Verification items for the finished model (mm, model axes). A direction names the side the tool comes from. Give positions to 0.01 mm unless a question says otherwise; leave off trailing zeros. Order: outer loops, then holes, each group sorted by start corner. A loop starts at its lowest first (then second) coordinate and runs counter-clockwise, first axis right, second up.
(1) Scan lines: L1, parallel to X at y = 16, z = -186; L2, parallel to Z at x = 152, y = 9.5; L3, parallel to Y at x = 197, z = -14. Record each from-to range of solid material in increasing order.
(2) Mould release check, pull along Y, two halves, no side actions. Record for faces 1 (the face through (44.071, 30, -186)), 2 (the face through (46.576, 52.068, -185.846)), 3 (the face through (67.531, 25.555, -11.772)): pulls with the +Y half, pulls with the -Y half, needs draft (parallel to the pull), parting line crosses it, or undercut.
(3) Gauge pin test, flat ends, axial feed: pin 1 (9.5 mm diameter, centred on y = 20.5, z = -8, fed in from +X); pin 2 (2 mm diameter, centred on x = 216, z = -131.5, fed in from +Y); pin 3 (6 mm diameter, centred on y = 42.545, z = -186.055, fed in from -X); pin 4 (1.5 mm diameter, centred on x = 122.5, y = 14, fed in from -Z). Record the tip position at first contact, or that the pin passes through.
(4) Sectioned sample at B-B on z = -138. Record the cut outline in (x, y).
(5) Access from +Z, -Z, +X, -X, +Y, -Y to the whole of each face (thin tool, end or side, straight path). Record for faces 4 (the face through (67.531, 33.018, -9.316)), 5 (the face through (70.106, 20, -9)), 6 (the face through (46.576, 41.28, -183.005)), 7 (the face through (153.672, 30, -186)), 8 (the face through (156.466, 20, -9)).
(6) Sectioned sample at A-A on x = 246.5. Record the cut outline in (y, z), plus the area to 3 significant figures.
```python
from build123d import *

# Parameters (mm, degrees)
SKETCH1_W               = 342.9
SKETCH1_H               = 195.58
BOSS_EXTRUDE1_DEPTH     = 7.62
SKETCH2_W               = 5.08
SKETCH2_H               = 19.05
BOSS_EXTRUDE2_DEPTH     = 25.4
SKETCH3_R               = 3.048
CUT_EXTRUDE1_DEPTH      = 309.353685576
SKETCH2_4_W             = 5.08
SKETCH2_4_H             = 19.05
SKETCH2_4_W_2           = 9.525
BOSS_EXTRUDE3_DEPTH     = 44.45
SKETCH4_R               = 3.302
CUT_EXTRUDE2_DEPTH      = 45.071314424
CUT_EXTRUDE2_DEPTH_BACK = 492.252


with BuildPart() as part:
    # Sketch1 → Boss-Extrude1 (new body)
    with BuildSketch(Plane(origin=(0, 0, 0), x_dir=(1, 0, 0), z_dir=(0, 1, 0))):
        with Locations((171.45, 97.79)):
            Rectangle(SKETCH1_W, SKETCH1_H)
    extrude(amount=BOSS_EXTRUDE1_DEPTH)

    # Sketch2 → Boss-Extrude2 (add)
    with BuildSketch(Plane(origin=(0, 7.62, 0), x_dir=(1, 0, 0), z_dir=(0, 1, 0))):
        with Locations((37.086314424, 9.525)):
            Rectangle(SKETCH2_W, SKETCH2_H)
        with Locations((67.566314424, 9.525)):
            Rectangle(SKETCH2_W, SKETCH2_H)
        with Locations((153.926314424, 9.525)):
            Rectangle(SKETCH2_W, SKETCH2_H)
        with Locations((123.446314424, 9.525)):
            Rectangle(SKETCH2_W, SKETCH2_H)
    extrude(amount=BOSS_EXTRUDE2_DEPTH)

    # Sketch3 → Cut-Extrude1 (cut, through all)
    with BuildSketch(Plane.ZY.offset(-34.546314424)):
        with Locations((-9.525, 23.495)):
            Circle(SKETCH3_R)
        with BuildLine():
            Line((-19.05, 23.495), (-20.422011891, 33.02))
            Line((-20.422011891, 33.02), (2.969055393, 35.880507904))
            Line((2.969055393, 35.880507904), (0, 23.495))
            ThreePointArc((0, 23.495), (-9.525, 33.02), (-19.05, 23.495))
        make_face()
    extrude(amount=-CUT_EXTRUDE1_DEPTH, mode=Mode.SUBTRACT)

    # Sketch2_4 → Boss-Extrude3 (add)
    with BuildSketch(Plane(origin=(0, 7.62, 0), x_dir=(1, 0, 0), z_dir=(0, 1, 0))):
        with Locations((46.611314424, 186.055)):
            Rectangle(SKETCH2_4_W, SKETCH2_4_H)
        with Locations((98.871814424, 186.055)):
            Rectangle(SKETCH2_4_W_2, SKETCH2_4_H)
        with Locations((151.132314424, 186.055)):
            Rectangle(SKETCH2_4_W, SKETCH2_4_H)
    extrude(amount=BOSS_EXTRUDE3_DEPTH)

    # Sketch4 → Cut-Extrude2 (cut, two sides)
    with BuildSketch(Plane.ZY.offset(-44.071314424)) as cut_extrude2_sk:
        with Locations((-186.055, 42.545)):
            Circle(SKETCH4_R)
        with BuildLine():
            Line((-195.58, 42.545), (-197.59428292, 55.074082425))
            Line((-197.59428292, 55.074082425), (-172.116639762, 54.451508438))
            Line((-172.116639762, 54.451508438), (-176.53, 42.545))
            ThreePointArc((-176.53, 42.545), (-186.055, 52.07), (-195.58, 42.545))
        make_face()
    extrude(amount=CUT_EXTRUDE2_DEPTH, mode=Mode.SUBTRACT)
    extrude(cut_extrude2_sk.sketch, amount=-CUT_EXTRUDE2_DEPTH_BACK, mode=Mode.SUBTRACT)


solid = part.part
```
Ans:
1. L1: x = 44.07 to 49.15, 94.11 to 103.63, 148.59 to 153.67
1. L2: z = -195.58 to -176.53, -19.05 to 0
1. L3: y = 0 to 7.62
2. face 1: needs draft
2. face 2: pulls with the +Y half
2. face 3: undercut
3. pin 1: stops at x = 156.47
3. pin 2: stops at y = 7.62
3. pin 3: passes through
3. pin 4: stops at z = -19.05
4. outline: (0, 0) - (342.9, 0) - (342.9, 7.62) - (0, 7.62) - close
5. face 4: +X, -X, +Y
5. face 5: +Z, -Z, +Y
5. face 6: +X, -X
5. face 7: -Z, +X, +Y
5. face 8: +Z, -Z, +X, +Y
6. outline: (0, -195.58) - (7.62, -195.58) - (7.62, 0) - (0, 0) - close
6. area: 1,490 mm2
